from build123d import *

# Parameters (mm, degrees)
F0_W     = 320
F0_H     = 145
F1_DEPTH = 45
F2_R     = 9.5
F2_R_2   = 6
F3_DEPTH = 5.5
F4_R     = 2
F5_DEPTH = 5
F7_R     = 8
F7_R_2   = 6
F8_DEPTH = 73.6875


# Not quite as in the source:
# - a pattern or mirror of a feature is missing from the dataset's text; its kind, count and spacing are read off the source's solid


with BuildPart() as f1:
    # F0 (on Front) → F1 (new body)
    with BuildSketch(Plane.XZ):
        with Locations((160, 0)):
            Rectangle(F0_W, F0_H)
    extrude(amount=F1_DEPTH)

    # F2 (on face) → F3 (join)
    with BuildSketch(Plane.XZ.offset(45)):
        with Locations((309, -40)):
            Circle(F2_R)
        with Locations((309, -40)):
            Circle(F2_R_2, mode=Mode.SUBTRACT)
        with Locations((309, 40)):
            Circle(F2_R)
        with Locations((309, 40)):
            Circle(F2_R_2, mode=Mode.SUBTRACT)
    extrude(amount=F3_DEPTH)

    # F4 (on face) → F5 (cut)
    with BuildSketch(Plane.XZ.offset(45)):
        with Locations((19, 62.5)):
            Circle(F4_R)
        with Locations((144, 62.5)):
            Circle(F4_R)
        with Locations((159, 62.5)):
            Circle(F4_R)
        with Locations((284, 62.5)):
            Circle(F4_R)
        with BuildLine():
            Line((24, 57.5), (14, 57.5))
            Line((14, 57.5), (14, 0))
            Line((14, 0), (14, -57.5))
            Line((14, -57.5), (24, -57.5))
            Line((24, -57.5), (24, -62.5))
            ThreePointArc((24, -62.5), (25.4644660941, -66.0355339059), (29, -67.5))
            Line((29, -67.5), (134, -67.5))
            ThreePointArc((134, -67.5), (137.5355339059, -66.0355339059), (139, -62.5))
            Line((139, -62.5), (139, -57.5))
            Line((139, -57.5), (164, -57.5))
            Line((164, -57.5), (164, -62.5))
            ThreePointArc((164, -62.5), (165.4644660941, -66.0355339059), (169, -67.5))
            Line((169, -67.5), (274, -67.5))
            ThreePointArc((274, -67.5), (277.5355339059, -66.0355339059), (279, -62.5))
            Line((279, -62.5), (279, -57.5))
            Line((279, -57.5), (289, -57.5))
            Line((289, -57.5), (289, 0))
            Line((289, 0), (289, 57.5))
            Line((289, 57.5), (279, 57.5))
            Line((279, 57.5), (279, 62.5))
            ThreePointArc((279, 62.5), (277.5355339059, 66.0355339059), (274, 67.5))
            Line((274, 67.5), (169, 67.5))
            ThreePointArc((169, 67.5), (165.4644660941, 66.0355339059), (164, 62.5))
            Line((164, 62.5), (164, 57.5))
            Line((164, 57.5), (139, 57.5))
            Line((139, 57.5), (139, 62.5))
            ThreePointArc((139, 62.5), (137.5355339059, 66.0355339059), (134, 67.5))
            Line((134, 67.5), (29, 67.5))
            ThreePointArc((29, 67.5), (25.4644660941, 66.0355339059), (24, 62.5))
            Line((24, 62.5), (24, 57.5))
        make_face()
        with Locations((284, -62.5)):
            Circle(F4_R)
        with Locations((159, -62.5)):
            Circle(F4_R)
        with Locations((144, -62.5)):
            Circle(F4_R)
        with Locations((19, -62.5)):
            Circle(F4_R)
    f5 = extrude(amount=-F5_DEPTH, mode=Mode.SUBTRACT)

    # F5_copies: F5 across plane
    add(f5.mirror(Plane.ZX.offset(-22.5)), mode=Mode.SUBTRACT)

    # F7 (on face) → F8 (join)
    with BuildSketch(Plane.XZ.offset(50.5)):
        with Locations((309, 40)):
            Circle(F7_R)
        with Locations((309, 40)):
            Circle(F7_R_2, mode=Mode.SUBTRACT)
    extrude(amount=F8_DEPTH)


solid = f1.part
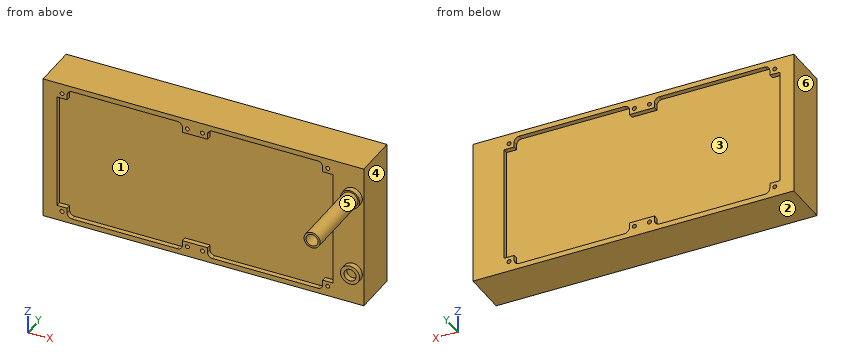
Work out the finished part from the listing and answer in its coordinate system (mm). Face numbers are marked on the shaded views. A direction names the side the tool comes from. Give positions to 0.01 mm unless a question says otherwise; leave off trailing zeros. Loops run counter-clockwise (first coordinate to the right, second up) from the corner with the lowest first, then second, coordinate; pieces in that order, holes last. Notation, with made-up numbers: (37, -22) - (63, -22) arc R16 ccw to (63, -6) - close; hole circle Ø2 at (-9, 88.5). An arc over 180 degrees is marked (long way). Answer in a Markdown table with one row per item. Add a question column.
Q1. Determine the mould class of the marked faces 1, 2, 3 and 4 for opening direction X: released by +X, released by -X, zero draft, split by the parting line, or undercut.
Q2. The part is cut by section A-A (x = 309). Determine the outline of the cut face in (y, z).
Q3. A tool of negligible diameter and unlimited length cuts with its end or side. For the marked faces 5 and 6, from which of +Z, -Z, +X, -X, +Y, -Y can it reach the whole face along a straight path? Write none if from no direction.
Q4. The part is cut by section D-D (x = 193). Determine the outline of the cut face in (y, z).
Q5. Each of these flat-tipped pins is pushed along its axis until it touches: P1, Ø4, axis at x = 73, z = -56.5, coming from the -Y side; P2, Ø6, axis at x = 280, z = -48, coming from the +Y side; P3, Ø3, axis at x = 158, z = 63.5, coming from the -Y side. Where does it stop, or does it pass through?
Q6. Consider line 1 along Z through (x, y) = (19, -3); line 2 along Y through (x, z) = (159, 47.5); line 3 along Y through (x, z) = (297, 12.5). Determine where each line is inside the solid, lowest interval first.
Q7. The part is cut by section B-B (z = 16). Determine the outline of the cut face in (x, y).
Q8. The part is cut by section C-C (y = -86). Determine the outline of the cut face in (x, z).
Solution:
| question | item | result |
|---|---|---|
| 1 | face 1 | undercut |
| 1 | face 2 | zero draft |
| 1 | face 3 | undercut |
| 1 | face 4 | released by +X |
| 2 | outline | (-124.19, 32) - (-50.5, 32) - (-50.5, 30.5) - (-45, 30.5) - (-45, -30.5) - (-50.5, -30.5) - (-50.5, -34) - (-45, -34) - (-45, -46) - (-50.5, -46) - (-50.5, -49.5) - (-45, -49.5) - (-45, -72.5) - (0, -72.5) - (0, 72.5) - (-45, 72.5) - (-45, 49.5) - (-50.5, 49.5) - (-50.5, 48) - (-124.19, 48) - (-124.19, 46) - (-45, 46) - (-45, 34) - (-124.19, 34) - close |
| 3 | face 5 | -Y |
| 3 | face 6 | +Z, -Z, -X, +Y, -Y |
| 4 | outline | (-45, -72.5) - (0, -72.5) - (0, -67.5) - (-5, -67.5) - (-5, 67.5) - (0, 67.5) - (0, 72.5) - (-45, 72.5) - (-45, 67.5) - (-40, 67.5) - (-40, -67.5) - (-45, -67.5) - close |
| 5 | P1 | stops at y = -40 |
| 5 | P2 | stops at y = -5 |
| 5 | P3 | stops at y = -45 |
| 6 | line 1 | z = -72.5 to -64.5, -60.5 to -57.5, 57.5 to 60.5, 64.5 to 72.5 |
| 6 | line 2 | y = -40 to -5 |
| 6 | line 3 | y = -45 to 0 |
| 7 | outline | (0, -45) - (14, -45) - (14, -40) - (289, -40) - (289, -45) - (320, -45) - (320, 0) - (289, 0) - (289, -5) - (14, -5) - (14, 0) - (0, 0) - close |
| 8 | outline | circle Ø16 at (309, 40); hole circle Ø12 at (309, 40) |
